Design review of the part built by this model. Coordinates are the model's own, in mm. Coordinates: 2 decimals unless noted, no trailing zeros. Loops run counter-clockwise (first coordinate to the right, second up) from the corner with the lowest first, then second, coordinate; pieces in that order, holes last.
Q1. For P1, Ø12, axis at y = -38.5, z = -220.5, coming from the +X side; P2, Ø4, axis at x = -42, y = -69, coming from the +Z side; P3, Ø2, axis at x = 200.5, y = -73.5, coming from the +Z side, all flat-tipped, find the tip position at first contact; note any pin that passes through.
Q2. Wall thickness on probe 1 along Z at (x, y) = (0, -62); probe 2 along Z at (x, y) = (0, -7); probe 3 along X at (y, z) = (-65.5, 58.5): over which ranges is each line inside the solid? List them lowest first.
Q3. Add section D-D on x = -247.5. Give the boundary of the cut face in (y, z).
Q4. Add section C-C on z = -201.5. Give the boundary of the cut face in (x, y).
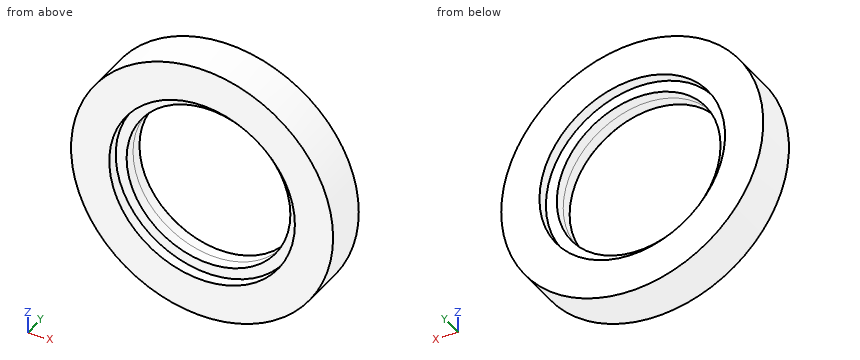
```python
from build123d import *

# Parameters (mm, degrees)
F0_R     = 304.8
F0_R_2   = 215.9
F1_DEPTH = 101.6
F3_R     = 224.342738
F3_R_2   = 190.498142
F4_DEPTH = 25.4
F5_R     = 221.566577
F5_R_2   = 190.5
F6_DEPTH = 25.4


with BuildPart() as f1:
    # F0 (on Front) → F1 (new body)
    with BuildSketch(Plane.XZ):
        Circle(F0_R)
        Circle(F0_R_2, mode=Mode.SUBTRACT)
    extrude(amount=F1_DEPTH)

    # F3 (on offset) → F4 (join)
    with BuildSketch(Plane.XZ.offset(50.8)):
        Circle(F3_R)
        Circle(F3_R_2, mode=Mode.SUBTRACT)
    extrude(amount=F4_DEPTH)

    # F5 (on face) → F6 (join)
    with BuildSketch(Plane(origin=(0, -50.8, 0), x_dir=(-1, 0, 0), z_dir=(0, 1, 0))):
        Circle(F5_R)
        Circle(F5_R_2, mode=Mode.SUBTRACT)
    extrude(amount=F6_DEPTH)


solid = f1.part
```
Entries:
1. P1: stops at x = 216.55
1. P2: stops at z = 302.16
1. P3: stops at z = 230.44
2. probe 1: z = -304.8 to -190.5, 190.5 to 304.8
2. probe 2: z = -304.8 to -215.9, 215.9 to 304.8
2. probe 3: x = -299.13 to -181.29, 181.29 to 299.13
3. outline: (-101.6, -177.9) - (0, -177.9) - (0, 177.9) - (-101.6, 177.9) - close
4. outline: (-228.69, -101.6) - (-77.53, -101.6) - (-77.53, -76.2) - (77.53, -76.2) - (77.53, -101.6) - (228.69, -101.6) - (228.69, 0) - (77.53, 0) - (77.53, -25.4) - (-77.53, -25.4) - (-77.53, 0) - (-228.69, 0) - close
